```python
from build123d import *

# Parameters (mm, degrees)
SKETCH1_R           = 12.5
BOSS_EXTRUDE1_DEPTH = 5
BOSS_EXTRUDE3_DEPTH = 10


with BuildPart() as part:
    # Sketch1 → Boss-Extrude1 (new body)
    with BuildSketch(Plane(origin=(0, 0, 0), x_dir=(1, 0, 0), z_dir=(0, 1, 0))):
        with Locations(Location((0, 0, 0), (0, 0, 270))):
            Circle(SKETCH1_R)
        Polygon((10.823922003, 0), (7.653668647, 7.653668647), (0, 10.823922003), (-7.653668647, 7.653668647), (-10.823922003, 0), (-7.653668647, -7.653668647), (0, -10.823922003), (7.653668647, -7.653668647), align=None, mode=Mode.SUBTRACT)
    extrude(amount=BOSS_EXTRUDE1_DEPTH)

    # Sketch2 → Boss-Extrude3 (add)
    with BuildSketch(Plane(origin=(0, 5, 0), x_dir=(1, 0, 0), z_dir=(0, 1, 0))):
        with BuildLine():
            Line((-8.340109868, -9.310884351), (-7.664468281, -7.67974127))
            ThreePointArc((-7.664468281, -7.67974127), (-10.026158107, 4.147125946), (0, 10.85))
            Line((0, 10.85), (0, 12.5))
            ThreePointArc((0, 12.5), (-11.675531131, 4.464523805), (-8.340109868, -9.310884351))
        make_face()
        with BuildLine():
            ThreePointArc((10.85, 0), (7.672108576, -7.672108576), (0, -10.85))
            Line((0, -10.85), (0, -12.5))
            ThreePointArc((0, -12.5), (8.838834765, -8.838834765), (12.5, 0))
            ThreePointArc((12.5, 0), (11.412549003, 5.099384792), (8.339403959, 9.311516612))
            Line((8.339403959, 9.311516612), (7.664457508, 7.679752021))
            ThreePointArc((7.664457508, 7.679752021), (10.02202235, 4.157110537), (10.85, 0))
        make_face()
    extrude(amount=BOSS_EXTRUDE3_DEPTH)


solid = part.part
```
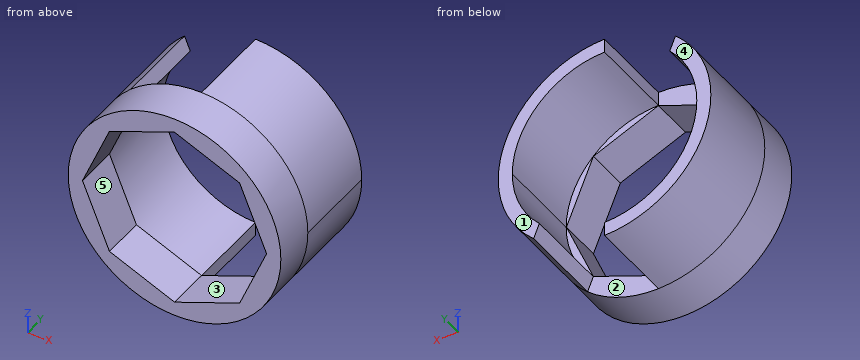
Could you check a few things on this model? Use its own coordinates, in mm. Face numbers are marked on the shaded views. A direction names the side the tool comes from. Coordinates: 2 decimals unless noted, no trailing zeros. Loops run counter-clockwise (first coordinate to the right, second up) from the corner with the lowest first, then second, coordinate; pieces in that order, holes last.
1) Thinking about a two-plate mould opening in X: for the marked faces 4 and 5, which applies, released by +X, released by -X, zero draft, split by the parting line, or undercut?
Reported:
face 4: zero draft
face 5: undercut
2) Imagine slicing it at D-D (x = 9). List the corners of the cut face in (y, z) for me.
Reported:
outline: (0, -8.67) - (15, -8.67) - (15, -6.06) - (5, -6.06) - (5, -4.4) - (0, -4.4) - close; (0, 4.4) - (5, 4.4) - (5, 6.06) - (15, 6.06) - (15, 8.67) - (0, 8.67) - close
3) Will these pins go through, and if not, where does the flat tip stop? pin 1 Ø3 at (x, y) = (-6, 13) entering from +Z; pin 2 Ø0.8 at (y, z) = (11, 11.5) entering from -X; pin 3 Ø4 at (x, y) = (4, 9) entering from +Z.
Reported:
pin 1: stops at z = -7.84
pin 2: stops at x = 0
pin 3: stops at z = 12.34
4) Imagine slicing it at A-A (y = 10.25). List the corners of the cut face in (x, z) for me.
Reported:
outline: (-8.34, 9.31) arc R12.5 ccw to (0, -12.5) - (0, -10.85) arc R10.85 cw to (-7.66, 7.68) - close; (0, 10.85) arc R10.85 cw to (7.66, -7.68) - (8.34, -9.31) arc R12.5 ccw to (0, 12.5) - close
5) Which directions (+Z, -Z, +X, -X, +Y, -Y) give clear straight access to the entire face, cutting with the end or side of a thin tool? Please do the marked faces 1, 2 and 3.
Reported:
face 1: +Z, -Z, +X, -X, +Y
face 2: +Y
face 3: +Y, -Y
6) Imagine slicing it at C-C (z = 9). List the corners of the cut face in (x, y) for me, and give its area (3 significant figures).
Reported:
outline: (-8.67, 0) - (-4.4, 0) - (-4.4, 5) - (-8.21, 5) - (-8.21, 15) - (-8.67, 15) - close; (4.4, 0) - (8.67, 0) - (8.67, 15) - (6.06, 15) - (6.06, 5) - (4.4, 5) - close
area: 73.5 mm2
7) Imagine slicing it at B-B (x = 3). List the corners of the cut face in (y, z) for me.
Reported:
outline: (0, -12.13) - (5, -12.13) - (5, -9.58) - (0, -9.58) - close; (0, 9.58) - (5, 9.58) - (5, 10.43) - (15, 10.43) - (15, 12.13) - (0, 12.13) - close
8) Please list where these lines run through material, in increasing order: line 1 along Y through (x, z) = (-10.75, -1); line 2 along Z through (x, y) = (-1.75, 4.75); line 3 along Z through (x, y) = (-8.5, 8.25).
Reported:
line 1: y = 0 to 5
line 2: z = -12.38 to -10.1, 10.1 to 12.38
line 3: z = -9.17 to -6.74, 6.74 to 9.17
